Input: part model. Units: mm. Frame: model coordinates. A direction names the side the tool comes from. Round coordinates to 2 decimals unless told otherwise and drop trailing zeros. Loops run counter-clockwise (first coordinate to the right, second up) from the corner with the lowest first, then second, coordinate; pieces in that order, holes last.
1) Section C-C, the plane z = 26. Return loops of the section in (x, y) (3 decimals), and give its area (3 significant figures).
2) Section A-A, the plane y = -21. Return loops of the section in (x, z).
3) Ray query, line 1 along Z through (x, y) = (-14, -16.75); line 2 along X through (y, z) = (-15.75, 10); line 3 along Y through (x, z) = (-9.5, 27.5). Return the intervals inside material, ascending.
4) First-contact query: pin 1 (8 mm diameter, centred on x = -16.5, z = -12.5, fed in from -Y); pin 2 (8 mm diameter, centred on x = 18.5, y = -6.5, fed in from +Z). Flat tips, straight axial feed; report the tip coordinate or a pass-through.
5) Access query for faces 1 (the face through (23.95, -3.46, 31.97)), 2 (the face through (-25, -25.4, 0)), 3 (the face through (0, -14, -34.46)). Directions: +Z, -Z, +X, -X, +Y, -Y. A direction counts if a zero-diameter tool reaches every point of the face in a straight line with its end or side. Return the directions, or none.
6) Draft query along X for faces 4 (the face through (-26, -13, -1)), 5 (the face through (24.447, -8.679, 23.395)), 6 (the face through (26, -13, -1)), 7 (the face through (0, -13, -37)). Return one class per face: pulls with the +X half, pulls with the -X half, needs draft (parallel to the pull), parting line crosses it, or undercut.
7) Section B-B, the plane x = -6. Return loops of the section in (y, z), and give its area (3 significant figures).
8) Section D-D, the plane z = -28.5. Return loops of the section in (x, y).
from build123d import *

# Parameters (mm, degrees)
F0_W     = 52
F0_H     = 74
F1_DEPTH = 25.4
F2_T     = -2.54
F4_D     = 15.24
F4_DEPTH = 12.7
F4_TIP   = 4.578557917


with BuildPart() as f1:
    # F0 (on Front) → F1 (new body)
    with BuildSketch(Plane.XZ):
        Rectangle(F0_W, F0_H)
    extrude(amount=F1_DEPTH)

    # F2
    f2_openings = [f1.faces().sort_by_distance(p)[0] for p in [
        (0, -25.4, 0),
    ]]
    offset(amount=F2_T, openings=f2_openings)

    # F4
    with Locations(Plane.XY.offset(37)):
        with Locations((-18.0935505778, -7.8645283356), (18.3343663812, -8.6078010499)):
            Hole(F4_D / 2, depth=F4_DEPTH)
            with Locations((0, 0, -(F4_DEPTH + F4_TIP / 2))):  # 118° drill point
                Cone(0, F4_D / 2, F4_TIP, mode=Mode.SUBTRACT)


solid = f1.part
Final values:
1. outline: (-26, -25.4) - (-23.46, -25.4) - (-23.46, -13.274) arc R7.62 cw (long way) to (-12.643, -2.54) - (13.725, -2.54) arc R7.62 cw to (22.944, -2.54) - (23.46, -2.54) - (23.46, -2.969) arc R7.62 cw to (23.46, -14.246) - (23.46, -25.4) - (26, -25.4) - (26, 0) - (-26, 0) - close
1. area: 185 mm2
2. outline: (-26, -37) - (26, -37) - (26, 37) - (-26, 37) - close; hole (-23.46, -34.46) - (23.46, -34.46) - (23.46, 34.46) - (-23.46, 34.46) - close
3. line 1: z = -37 to -34.46, 34.46 to 37
3. line 2: x = -26 to -23.46, 23.46 to 26
3. line 3: y = -2.54 to 0
4. pin 1: stops at y = -2.54
4. pin 2: stops at z = 23.4
5. face 1: +Z
5. face 2: +Z, -Z, +X, -X, -Y
5. face 3: -Y
6. face 4: pulls with the -X half
6. face 5: undercut
6. face 6: pulls with the +X half
6. face 7: needs draft
7. outline: (-25.4, -37) - (0, -37) - (0, 37) - (-25.4, 37) - (-25.4, 34.46) - (-2.54, 34.46) - (-2.54, -34.46) - (-25.4, -34.46) - close
7. area: 304 mm2
8. outline: (-26, -25.4) - (-23.46, -25.4) - (-23.46, -2.54) - (23.46, -2.54) - (23.46, -25.4) - (26, -25.4) - (26, 0) - (-26, 0) - close
